from build123d import *

# Parameters (mm, degrees)
F2_W     = 40.64
F2_H     = 30.48
F3_DEPTH = 101.6
F4_SIZE  = 25.4


with BuildPart() as f1:
    # F0 (on Top) → F1 (revolve)
    with BuildSketch(Plane.XY):
        with BuildLine():
            Line((0, -50.8), (0, 50.8))
            ThreePointArc((0, 50.8), (-50.8, 0), (0, -50.8))
        make_face()
    revolve(axis=Axis((0, 0, 0), (0, -1, 0)))

    # F2 (on Top) → F3 (join)
    with BuildSketch(Plane.XY):
        with Locations((20.32, 15.24)):
            Rectangle(F2_W, F2_H)
    extrude(amount=F3_DEPTH)

    # F4
    f4_edges = [f1.edges().sort_by_distance(p)[0] for p in [
        (20.32, 0, 101.6),
    ]]
    chamfer(f4_edges, length=F4_SIZE)


solid = f1.part
Input: part model. Units: mm. Frame: model coordinates. A direction names the side the tool comes from. Coordinates: 2 decimals unless noted, no trailing zeros. Loops run counter-clockwise (first coordinate to the right, second up) from the corner with the lowest first, then second, coordinate; pieces in that order, holes last. Notation, with made-up numbers: (-4, -23) -> (26, -23) arc R23 ccw to (26, 16) -> close; hole circle Ø10 at (39.25, -20.5). An arc over 180 degrees is marked (long way). One line per item, written item: value.
(1) Cut plane A-A (x = 10.5). Output: boundary loops of the cut face in (y, z), then the cut area to 3 significant figures.
Answer below:
outline: (0, 49.7) arc R49.7 ccw (long way) to (30.48, 39.26) -> (30.48, 101.6) -> (25.4, 101.6) -> (0, 76.2) -> close
area: 9,120 mm2
(2) Cut plane C-C (z = -31.5). Output: boundary loops of the cut face in (x, y).
Answer below:
outline: circle Ø79.71 at (0, 0)
(3) Cut plane D-D (y = -14.5). Output: boundary loops of the cut face in (x, z).
Answer below:
outline: circle Ø97.37 at (0, 0)
(4) Ray query, line 1 along Y through (x, z) = (2, 73); line 2 along X through (y, z) = (27, 77); line 3 along Z through (x, y) = (-3, -20). Return the intervals inside material, ascending.
Answer below:
line 1: y = 0 to 30.48
line 2: x = 0 to 40.64
line 3: z = -46.6 to 46.6
(5) Cut plane B-B (y = 13.5). Output: boundary loops of the cut face in (x, z).
Answer below:
outline: (0, 48.97) arc R48.97 ccw (long way) to (40.64, 27.33) -> (40.64, 89.7) -> (0, 89.7) -> close
(6) Set-up query: faces 1 (the face through (20, 28, 101.6)), 2 (the face through (20, 12.5, 88.7)), 3 (the face through (20, 0, 58)), 4 (the face through (0, 18, 71)), 5 (the face through (20, 30.48, 61)). Return all of +Z, -Z, +X, -X, +Y, -Y with unobstructed straight access to the full face (end or side cutting, diameter ignored); none if empty.
Answer below:
face 1: +Z, +X, -X, +Y, -Y
face 2: +Z, +X, -X, -Y
face 3: +Z, +X, -Y
face 4: +Z, -X, +Y
face 5: +Z, +X, +Y
(7) Pin query (flat end, axial travel): pin 1 Ø1.5 at (x, z) = (28.5, 79) entering from +Y; pin 2 Ø1.5 at (x, z) = (20.5, 9.5) entering from +Y; pin 3 Ø1 at (x, y) = (-20.5, -26.5) entering from -Z. Return the tip coordinate at first contact, or that it passes through.
Answer below:
pin 1: stops at y = 30.48
pin 2: stops at y = 45.86
pin 3: stops at z = -38.62
